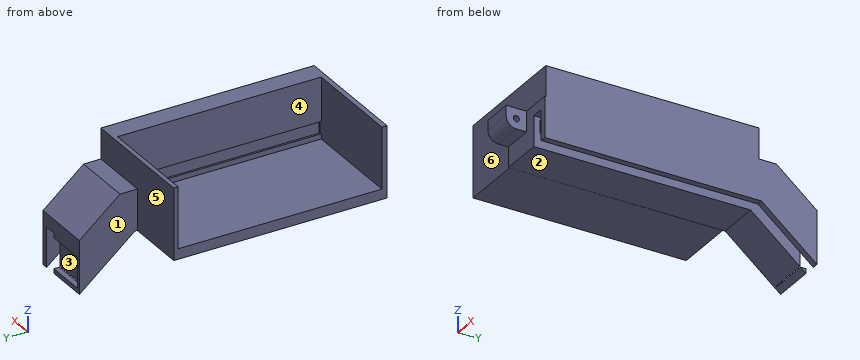
```python
from build123d import *

# Parameters (mm, degrees)
SKETCH_1_W           = 30
SKETCH_1_H           = 20
SKETCH_16_W          = 6
SKETCH_16_H          = 15
SKETCH_20_W          = 44.009262039
SKETCH_20_H          = 100
ARDUINO_DEPTH        = 15
SKETCH_36_W          = 15
SKETCH_36_H          = 10
EXTRUDE_1_DEPTH      = 10
CUT_EXTRUDE_25_DEPTH = 15
CUT_EXTRUDE_28_DEPTH = 30
SKETCH_41_W          = 19.503659652
SKETCH_41_H          = 15
CUT_EXTRUDE_29_DEPTH = 3
EXTRUDE_2_DEPTH      = 30
SKETCH_46_W          = 30
SKETCH_46_H          = 100
CUT_EXTRUDE_31_DEPTH = 15
EXTRUDE_3_DEPTH      = 15
SKETCH_48_W          = 6
SKETCH_48_H          = 100
CUT_EXTRUDE_32_DEPTH = 5
SKETCH_49_R          = 1.5
CUT_EXTRUDE_33_DEPTH = 15


with BuildPart() as part:
    # 扫描1: sweep along a path in 草图2
    with BuildLine(Plane(origin=(-2.57, 0, 0), x_dir=(0, 0, -1), z_dir=(1, 0, 0))) as sweep_1_path:
        Line((-5.367132867, 0), (-5.367132867, 110))
        Line((-5.367132867, 110), (19.805856068, 140))
    # 草图1 → 扫描1 (sweep)
    with BuildSketch(Plane(origin=(0, 0, 0), x_dir=(1, 0, 0), z_dir=(0, 1, 0))):
        with Locations((-2.56993007, -5.367132867)):
            Rectangle(SKETCH_1_W, SKETCH_1_H)
    sweep(path=sweep_1_path.line, transition=Transition.RIGHT)

    # 切除-扫描2: sweep along a path in 草图19
    with BuildLine(Plane(origin=(6.43006993, 0, 0), x_dir=(0, 0, -1), z_dir=(1, 0, 0))) as sweep_2_path:
        Line((21.720967176, 138.393030976), (-2.867132867, 109.090074414))
        Line((-2.867132867, 109.090074414), (-2.867132867, 0))
    # 草图16 → 切除-扫描2 (sweep, cut)
    with BuildSketch(Plane(origin=(0, 91.907852742, -77.119845338), x_dir=(1, 0, 0), z_dir=(0, 0.7660444431189769, -0.6427876096865407))):
        with Locations((6.43006993, -72.318099374)):
            Rectangle(SKETCH_16_W, SKETCH_16_H)
    sweep(path=sweep_2_path.line, transition=Transition.RIGHT, mode=Mode.SUBTRACT)

    # 草图20 → arduino (cut)
    with BuildSketch(Plane.XY.offset(15.367132867)):
        with Locations((-19.57456109, 53)):
            Rectangle(SKETCH_20_W, SKETCH_20_H)
    extrude(amount=-ARDUINO_DEPTH, mode=Mode.SUBTRACT)

    # 草图36 → 凸台-拉伸1 (add)
    with BuildSketch(Plane.XZ):
        with Locations((-10.06993007, 10.367132867)):
            Rectangle(SKETCH_36_W, SKETCH_36_H)
    extrude(amount=EXTRUDE_1_DEPTH)

    # 草图37 → 切除-拉伸25 (cut)
    with BuildSketch(Plane.ZY.offset(17.56993007)):
        with BuildLine():
            Line((5.367132867, -10), (5.367132867, -5))
            ThreePointArc((5.367132867, -5), (6.831598961, -8.535533906), (10.367132867, -10))
            Line((10.367132867, -10), (5.367132867, -10))
        make_face()
    extrude(amount=-CUT_EXTRUDE_25_DEPTH, mode=Mode.SUBTRACT)

    # 草图40 → 切除-拉伸28 (cut)
    with BuildSketch(Plane.ZY.offset(17.56993007)):
        Polygon((-27.466300499, 133.572123903), (-1.358154713, 133.572123903), (-12.145411637, 146.427876097), align=None)
    extrude(amount=-CUT_EXTRUDE_28_DEPTH, mode=Mode.SUBTRACT)

    # 草图41 → 切除-拉伸29 (cut)
    with BuildSketch(Plane(origin=(0, 133.572123903, 0), x_dir=(1, 0, 0), z_dir=(0, 1, 0))):
        with Locations((-6.321759896, 17.716300499)):
            Rectangle(SKETCH_41_W, SKETCH_41_H)
    extrude(amount=-CUT_EXTRUDE_29_DEPTH, mode=Mode.SUBTRACT)

    # 草图42 → 凸台-拉伸2 (add)
    with BuildSketch(Plane.ZY.offset(17.56993007)):
        Polygon((-4.730811685, 105.128164413), (-4.632867133, 0.51377094), (15.367132867, 0.51377094), (15.367132867, 105.128164413), align=None)
    extrude(amount=EXTRUDE_2_DEPTH)

    # 草图46 → 切除-拉伸31 (cut)
    with BuildSketch(Plane.XY.offset(15.367132867)):
        with Locations((-32.56993007, 53)):
            Rectangle(SKETCH_46_W, SKETCH_46_H)
    extrude(amount=-CUT_EXTRUDE_31_DEPTH, mode=Mode.SUBTRACT)

    # 草图47 → 凸台-拉伸3 (add)
    with BuildSketch(Plane.XY.offset(15.367132867)):
        Polygon((-47.56993007, 105.128164413), (-47.56993007, 103), (2.43006993, 103), (2.43006993, 3), (-47.56993007, 3), (-47.56993007, 0.51377094), (12.43006993, 0.51377094), (12.43006993, 105.128164413), align=None)
    extrude(amount=EXTRUDE_3_DEPTH)

    # 草图48 → 切除-拉伸32 (cut)
    with BuildSketch(Plane.ZY.offset(-2.43006993)):
        with Locations((5.88172197, 53)):
            Rectangle(SKETCH_48_W, SKETCH_48_H)
    extrude(amount=-CUT_EXTRUDE_32_DEPTH, mode=Mode.SUBTRACT)

    # 草图49 → 切除-拉伸33 (cut)
    with BuildSketch(Plane.ZY.offset(17.56993007)):
        with Locations((10.367132867, -5)):
            Circle(SKETCH_49_R)
    extrude(amount=-CUT_EXTRUDE_33_DEPTH, mode=Mode.SUBTRACT)


solid = part.part
```
Build history of the part. All positions in model axes, mm. Face numbers are marked on the shaded views. A direction names the side the tool comes from. Coordinates: 2 decimals unless noted, no trailing zeros. Write each loop counter-clockwise with the first axis right and the second up, starting at its lowest first coordinate (ties: lowest second). Pieces come first, ordered by that corner, then holes.
1. Band-saw the part on A-A, the plane x = -7. Give the cut face in (y, z).
Answer block:
outline: (-10, 10.37) arc R5 ccw to (-5, 5.37) - (0, 5.37) - (0, -4.63) - (106.36, -4.63) - (130.57, -24.95) - (130.57, -10.22) - (133.57, -10.22) - (133.57, -1.36) - (113.64, 15.37) - (105.13, 15.37) - (105.13, 30.37) - (103, 30.37) - (103, 0.37) - (3, 0.37) - (3, 30.37) - (0.51, 30.37) - (0.51, 15.37) - (-10, 15.37) - close; (130.89, -25.22) - (133.57, -27.47) - (133.57, -25.22) - close; hole circle Ø3 at (-5, 10.37)
2. Band-saw the part on B-B, the plane z = -18. Give the cut face in (x, y).
Answer block:
outline: (-17.57, 122.29) - (3.43, 122.29) - (3.43, 130.57) - (-16.07, 130.57) - (-16.07, 133.57) - (-17.57, 133.57) - close; (9.43, 122.29) - (12.43, 122.29) - (12.43, 133.57) - (9.43, 133.57) - close
3. Drop flat-ended pins along their axis: pin 1 (2.5 mm diameter, centred on x = 11, y = 60.5, fed in from -Z); pin 2 (8 mm diameter, centred on x = -24.5, z = 15.5, fed in from -Y); pin 3 (0.8 mm diameter, centred on x = -9, y = 131.5, fed in from +Z). Give the stop position or say it passes through.
Answer block:
pin 1: stops at z = -4.63
pin 2: stops at y = 0.51
pin 3: stops at z = 0.72
4. Band-saw the part on C-C, the plane y = 70.5. Give the cut face in (x, z), and give its area (3 significant figures).
Answer block:
outline: (-47.57, -4.7) - (-17.57, -4.7) - (-17.57, -4.63) - (3.43, -4.63) - (3.43, 2.88) - (2.43, 2.88) - (2.43, 0.37) - (-47.57, 0.37) - close; (2.43, 8.88) - (3.43, 8.88) - (3.43, 10.37) - (9.43, 10.37) - (9.43, -4.63) - (12.43, -4.63) - (12.43, 30.37) - (2.43, 30.37) - close
area: 506 mm2
5. 3-axis set-ups, long thin cutter, end or side, ignore diameter. For the marked faces 4, 5 and 6: which of +Z, -Z, +X, -X, +Y, -Y reach the whole face in a straight line?
Answer block:
face 4: +Z, -X
face 5: +Z, -X, +Y
face 6: +Z, -X, -Y
6. Band-saw the part on D-D, the plane x = -34. Give the cut face in (y, z).
Answer block:
outline: (0.51, -4.63) - (105.13, -4.73) - (105.13, 30.37) - (103, 30.37) - (103, 0.37) - (3, 0.37) - (3, 30.37) - (0.51, 30.37) - close
7. Drill centre lines: probe 1 along Z at (x, y) = (3, 21.5); probe 2 along Y at (x, z) = (-11.5, 25); probe 3 along X at (y, z) = (57, -1). Where is each one in solid material? Low to high.
Answer block:
probe 1: z = -4.63 to 2.88, 8.88 to 30.37
probe 2: y = 0.51 to 3, 103 to 105.13
probe 3: x = -47.57 to 3.43, 9.43 to 12.43
8. Pull direction X, two halves, no side cores. Call the marked faces 1, 2 and 3: released by +X, released by -X, zero draft, split by the parting line, or undercut.
Answer block:
face 1: released by -X
face 2: zero draft
face 3: undercut
